Can you work these out from the drawing? Everything is in mm from the part's minimum corner. A direction names the side the tool comes from. Coordinates: 2 decimals unless noted, no trailing zeros. Order: outer loops, then holes, each group sorted by start corner. A loop starts at its lowest first (then second) coordinate and runs counter-clockwise, first axis right, second up. Notation, with made-up numbers: (18.5, 47) - (45.5, 47) arc R16 ccw to (45.5, 67) - close; hole circle Ø8 at (59, 16.5). An arc over 180 degrees is marked (long way). Answer as CSV lines item,"result". Start each with the question number.
Q1. Suppose I cut it at D-D (x = 14.5). Please give me the cut outline in (y, z) (1 decimal).
Q2. Thinking about a two-plate mould opening in X: for the marked faces 3, 4 and 5, which applies, released by +X, released by -X, zero draft, split by the parting line, or undercut?
Q3. Suppose I cut it at B-B (z = 8). Please give me the cut outline in (x, y) (1 decimal), then the cut area to 3 significant figures.
Q4. For pin 1 Ø1.8 at (x, z) = (1, 7) entering from -Y; pin 2 Ø7 at (x, z) = (44, 6) entering from -Y; pin 3 Ø6 at (y, z) = (4, 4) entering from +X (1 decimal), each with a flat end and sliding along its axis, tell me the tip position at first contact or that it passes through.
Q5. Suppose I cut it at A-A (z = 3.25). Please give me the cut outline in (x, y) (1 decimal), then the cut area to 3 significant figures.
Q6. Suppose I cut it at C-C (x = 48). Please give me the cut outline in (y, z) (1 decimal).
Q7. For the marked faces 1 and 2, which set-ups out of +Z, -Z, +X, -X, +Y, -Y let a thin tool reach every point of the face, with its end or its side?
Q8. I need wall thicknesses on line 1 (Y direction, x = 34, z = 7); line 2 (Y direction, x = 31.5, z = 8.75); line 3 (X direction, y = 13, z = 12) (1 decimal). Which ranges of each line are inside material? Lowest first, please.
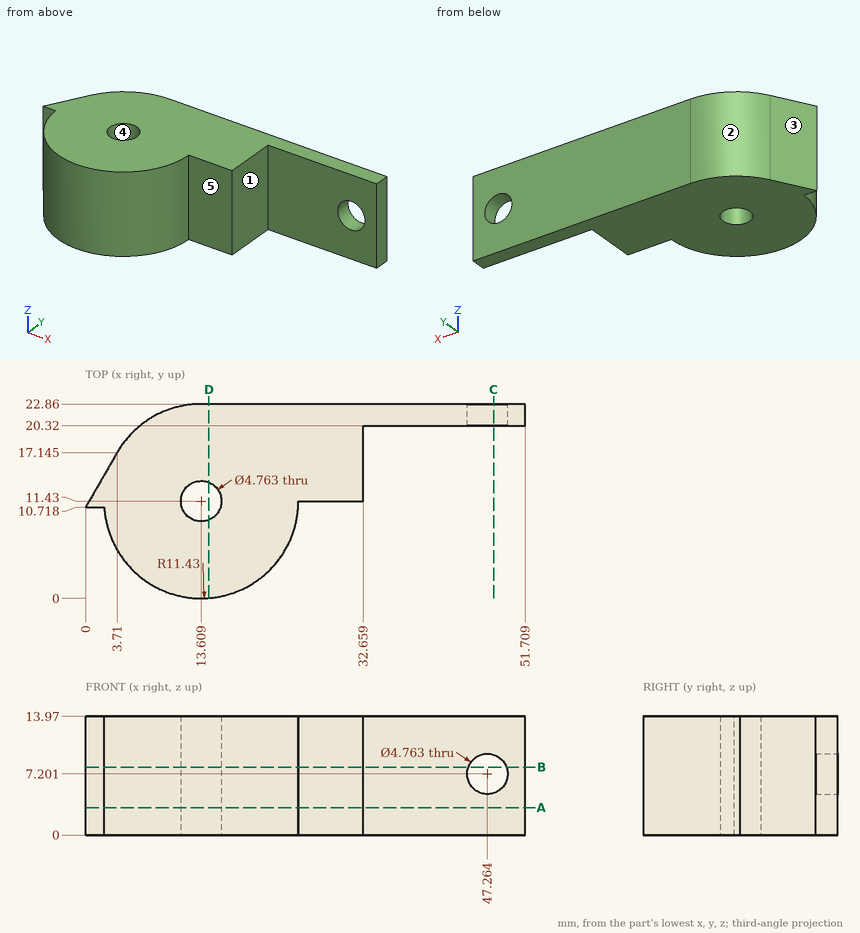
Here are the results:
1,outline,"(0, 0) - (9.2, 0) - (9.2, 14) - (0, 14) - close; (13.6, 0) - (22.9, 0) - (22.9, 14) - (13.6, 14) - close"
2,face 3,"released by -X"
2,face 4,"undercut"
2,face 5,"zero draft"
3,outline,"(0, 10.7) - (2.2, 10.7) arc R11.4 ccw to (25, 11.4) - (32.7, 11.4) - (32.7, 20.3) - (45, 20.3) - (45, 22.9) - (13.6, 22.9) arc R11.4 ccw to (3.7, 17.1) - close; (49.5, 20.3) - (51.7, 20.3) - (51.7, 22.9) - (49.5, 22.9) - close; hole circle Ø4.8 at (13.6, 11.4)"
3,area,"550 mm²"
4,pin 1,"stops at y = 10.72"
4,pin 2,"stops at y = 20.32"
4,pin 3,"stops at x = 24.1"
5,outline,"(0, 10.7) - (2.2, 10.7) arc R11.4 ccw to (25, 11.4) - (32.7, 11.4) - (32.7, 20.3) - (51.7, 20.3) - (51.7, 22.9) - (13.6, 22.9) arc R11.4 ccw to (3.7, 17.1) - close; hole circle Ø4.8 at (13.6, 11.4)"
5,area,"561 mm²"
6,outline,"(20.3, 0) - (22.9, 0) - (22.9, 4.9) - (20.3, 4.9) - close; (20.3, 9.5) - (22.9, 9.5) - (22.9, 14) - (20.3, 14) - close"
7,face 1,"+Z, -Z, +X, -Y"
7,face 2,"+Z, -Z, -X, +Y"
8,line 1,"y = 20.32 to 22.86"
8,line 2,"y = 11.43 to 22.86"
8,line 3,"x = 1.3 to 11.8, 15.4 to 32.7"
